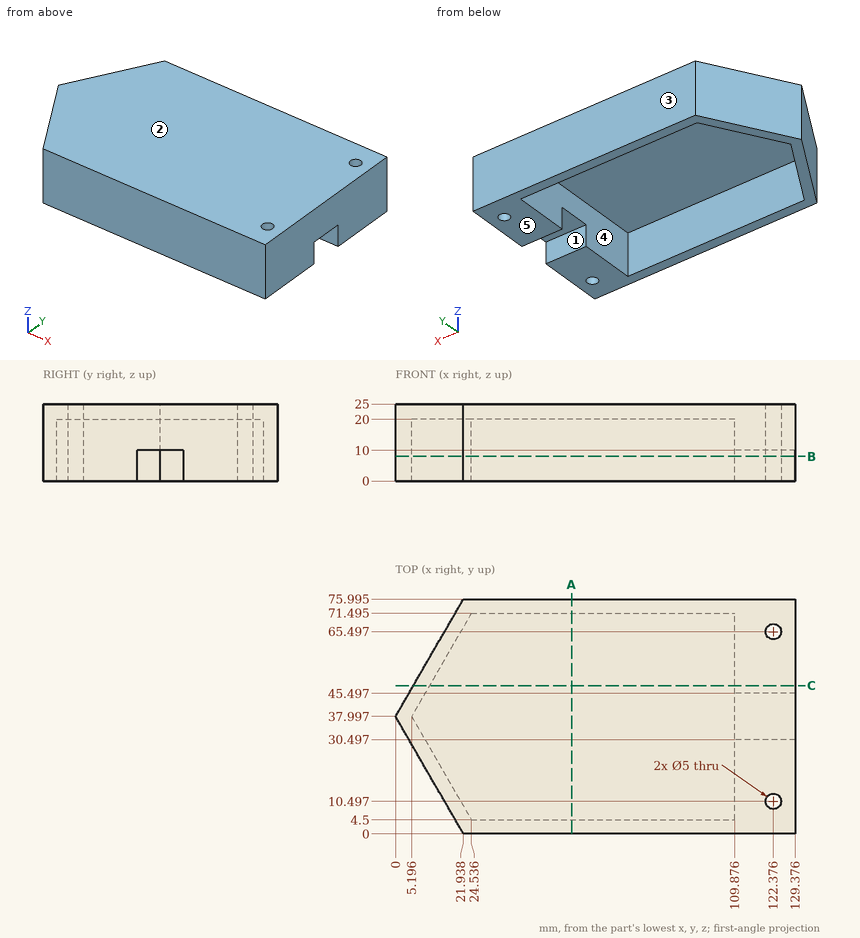
Verification items for this drawing (mm, ordinates from the low corner). A direction names the side the tool comes from. Give positions to 0.01 mm unless a question says otherwise; leave off trailing zeros. Write each loop counter-clockwise with the first axis right and the second up, starting at its lowest first coordinate (ties: lowest second). Pieces come first, ordered by that corner, then holes. Notation, with made-up numbers: (67.25, 80.25) -> (116.25, 80.25) arc R35 ccw to (116.25, 118.25) -> close; hole circle Ø6 at (43.5, 3.25). An arc over 180 degrees is marked (long way). Use CSV: the item, a comma, the result in double quotes.
(1) Sectioned sample at B-B (z = 8). Record the cut outline in (x, y) (1 decimal), plus the area to 3 significant figures.
Derived:
outline,"(0, 38) -> (21.9, 0) -> (129.4, 0) -> (129.4, 30.5) -> (109.9, 30.5) -> (109.9, 4.5) -> (24.5, 4.5) -> (5.2, 38) -> (24.5, 71.5) -> (109.9, 71.5) -> (109.9, 45.5) -> (129.4, 45.5) -> (129.4, 76) -> (21.9, 76) -> close; hole circle Ø5 at (122.4, 10.5); hole circle Ø5 at (122.4, 65.5)"
area,"2,300 mm^2"
(2) Release check for a two-part mould opening along Y. For the marked faces 1, 2 and 3 record: +Y half, -Y half, draft (parallel to the pull), parting line (faces both ways), or undercut.
Derived:
face 1,"undercut"
face 2,"draft"
face 3,"+Y half"
(3) Go/stop test with flat-tipped pins: pin 1 (20 mm diameter, centred on x = 83.5, y = 54.5, fed in from -Z); pin 2 (6 mm diameter, centred on x = 68.5, z = 5.5, fed in from -Y); pin 3 (12 mm diameter, centred on x = 118, y = 37.5, fed in from -Z); pin 4 (1 mm diameter, centred on y = 13, z = 9.5, fed in from -X). Record where each tip stops, or that it passes through.
Derived:
pin 1,"stops at z = 20"
pin 2,"stops at y = 0"
pin 3,"stops at z = 10"
pin 4,"stops at x = 14.14"
(4) Material ranges on L1, parallel to Y at x = 89.5, z = 12 (1 decimal); L2, parallel to Y at x = 114, z = 6.25 (1 decimal); L3, parallel to X at y = 65, z = 8.25 (1 decimal), recorded low to high.
Derived:
L1,"y = 0 to 4.5, 71.5 to 76"
L2,"y = 0 to 30.5, 45.5 to 76"
L3,"x = 15.6 to 20.8, 109.9 to 119.9, 124.8 to 129.4"
(5) Sectioned sample at A-A (x = 57). Record the cut outline in (y, z) (1 decimal).
Derived:
outline,"(0, 0) -> (4.5, 0) -> (4.5, 20) -> (71.5, 20) -> (71.5, 0) -> (76, 0) -> (76, 25) -> (0, 25) -> close"
(6) Set-up check for the marked faces 4 and 5: record each of +Z, -Z, +X, -X, +Y, -Y from which the full face is reachable in a straight line by a thin tool's end or side.
Derived:
face 4,"-Z"
face 5,"-Z, +X, -X, +Y, -Y"
(7) Sectioned sample at C-C (y = 48). Record the cut outline in (x, z) (1 decimal).
Derived:
outline,"(5.8, 0) -> (11, 0) -> (11, 20) -> (109.9, 20) -> (109.9, 0) -> (129.4, 0) -> (129.4, 25) -> (5.8, 25) -> close"
